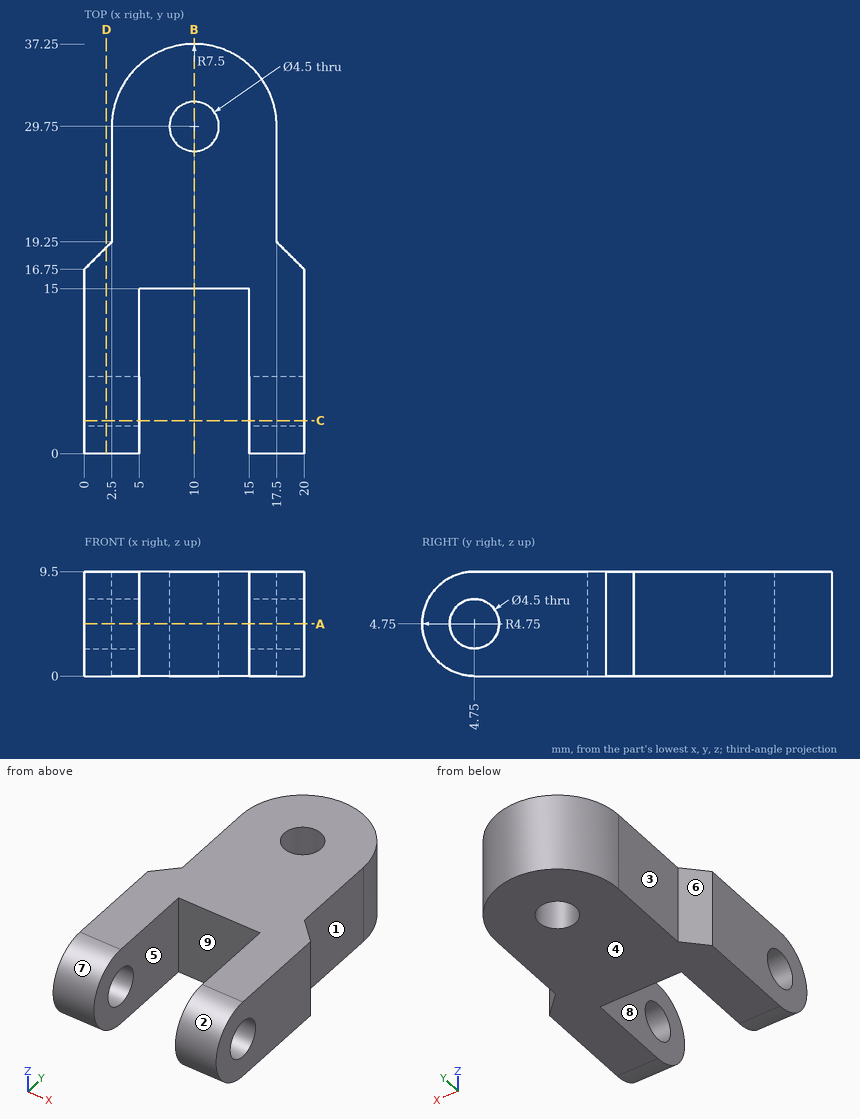
Could you check a few things on this drawing? It's one solid part, dimensions in mm from its lowest x, y, z. A direction names the side the tool comes from. Round coordinates to 2 decimals unless told otherwise and drop trailing zeros. Loops run counter-clockwise (first coordinate to the right, second up) from the corner with the lowest first, then second, coordinate; pieces in that order, holes last. Notation, with made-up numbers: (19, 7) -> (49, 7) arc R21 ccw to (49, 18) -> close; hole circle Ø2 at (-11, -8.75). An arc over 180 degrees is marked (long way). One line per item, written item: value. Start each with the question number.
1. For the marked faces 1, 2, 3, 4 and 5, which set-ups out of +Z, -Z, +X, -X, +Y, -Y let a thin tool reach every point of the face, with its end or its side?
2. If we section it at A-A, the plane z = 4.75: Write out the boundary of the cut face in (x, y).
3. If I drill on probe 1 along Y at (x, z) = (10, 4.75); probe 2 along Z at (x, y) = (18.9, 4.75); probe 3 along X at (y, z) = (14.5, 5), over which ranges is the centre line in solid material (lowest first)?
4. If we section it at C-C, the plane y = 3: Write out the boundary of the cut face in (x, z).
5. If we mould it in two halves opening along X, with no side actions, what happens to the marked faces 6, 7, 8 and 9? For each: pulls with the +X half, pulls with the -X half, needs draft (parallel to the pull), parting line crosses it, or undercut.
6. For pin 1 (6 mm diameter, centred on x = 16, y = 12.5, fed in from -Z); pin 2 (4 mm diameter, centred on y = 4.75, z = 4.75, fed in from +X); pin 3 (5 mm diameter, centred on x = 10, z = 2.5, fed in from -Y); pin 4 (5 mm diameter, centred on y = 23.5, z = 3.5, fed in from -X), each with a flat end and sliding along its axis, tell me the tip position at first contact or that it passes through.
7. If we section it at D-D, the plane x = 2: Write out the boundary of the cut face in (y, z).
8. If we section it at B-B, the plane x = 10: Write out the boundary of the cut face in (y, z), then the cut area to 3 significant figures.
Calculated:
1. face 1: +Z, -Z, +X, +Y
1. face 2: +X, -X, -Y
1. face 3: +Z, -Z, -X, +Y
1. face 4: -Z, +X, -X, +Y, -Y
1. face 5: +Z, -Z, -Y
2. outline: (0, 0) -> (5, 0) -> (5, 2.5) -> (0, 2.5) -> close; (0, 7) -> (5, 7) -> (5, 15) -> (15, 15) -> (15, 7) -> (20, 7) -> (20, 16.75) -> (17.5, 19.25) -> (17.5, 29.75) arc R7.5 ccw to (2.5, 29.75) -> (2.5, 19.25) -> (0, 16.75) -> close; (15, 0) -> (20, 0) -> (20, 2.5) -> (15, 2.5) -> close; hole circle Ø4.5 at (10, 29.75)
3. probe 1: y = 15 to 27.5, 32 to 37.25
3. probe 2: z = 0 to 2.5, 7 to 9.5
3. probe 3: x = 0 to 5, 15 to 20
4. outline: (0, 0.33) -> (5, 0.33) -> (5, 3.34) -> (0, 3.34) -> close; (0, 6.16) -> (5, 6.16) -> (5, 9.17) -> (0, 9.17) -> close; (15, 0.33) -> (20, 0.33) -> (20, 3.34) -> (15, 3.34) -> close; (15, 6.16) -> (20, 6.16) -> (20, 9.17) -> (15, 9.17) -> close
5. face 6: pulls with the -X half
5. face 7: needs draft
5. face 8: undercut
5. face 9: undercut
6. pin 1: stops at z = 0
6. pin 2: passes through
6. pin 3: stops at y = 15
6. pin 4: stops at x = 2.5
7. outline: (4.75, 0) -> (18.75, 0) -> (18.75, 9.5) -> (4.75, 9.5) arc R4.75 ccw to start; hole circle Ø4.5 at (4.75, 4.75)
8. outline: (15, 0) -> (27.5, 0) -> (27.5, 9.5) -> (15, 9.5) -> close; (32, 0) -> (37.25, 0) -> (37.25, 9.5) -> (32, 9.5) -> close
8. area: 169 mm²
